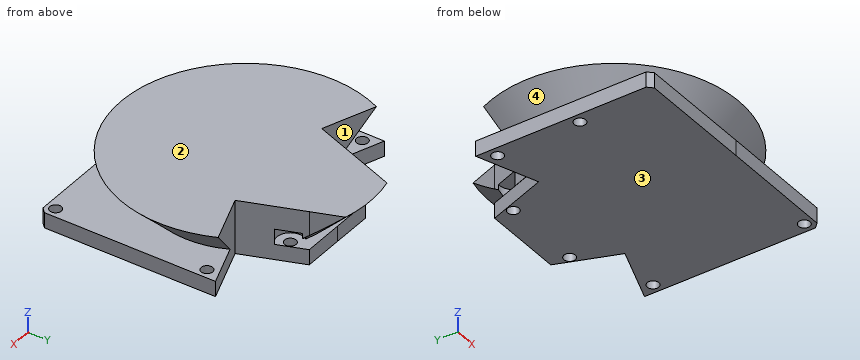
```python
from build123d import *

# Parameters (mm, degrees)
SKETCH9_R           = 1.4986
BOSS_EXTRUDE2_DEPTH = 4
SKETCH10_R          = 22.5
BOSS_EXTRUDE3_DEPTH = 10
BOSS_EXTRUDE3_DRAFT = -45
CUT_EXTRUDE1_DEPTH  = 10
SKETCH12_R          = 3.4986
CUT_EXTRUDE2_DEPTH  = 4


with BuildPart() as part:
    # Sketch9 → Boss-Extrude2 (new body)
    with BuildSketch(Plane.XY):
        Polygon((0, 45.894331692), (15.488494665, 40.257085472), (21.11579715, 55.718259441), (31.638563481, 55.718259441), (42.161245631, 55.760350338), (47.850347546, 40.321809178), (63.316169409, 46.020964031), (63.494666021, 1.396989332), (62.229756161, 0.121919512), (31.75, 0), (1.27, 0), (0, 1.27), align=None)
        with Locations((60.94984, 2.54)):
            Circle(SKETCH9_R, mode=Mode.SUBTRACT)
        with Locations((21.082, 50.8)):
            Circle(SKETCH9_R, mode=Mode.SUBTRACT)
        with Locations((2.54, 41.91)):
            Circle(SKETCH9_R, mode=Mode.SUBTRACT)
        with Locations(Location((60.792126991, 42.026504254, 0), (0, 0, 180))):
            Circle(SKETCH9_R, mode=Mode.SUBTRACT)
        with Locations(Location((42.214715469, 50.842265431, 0), (0, 0, 180))):
            Circle(SKETCH9_R, mode=Mode.SUBTRACT)
        with Locations((2.45872, 20.32)):
            Circle(SKETCH9_R, mode=Mode.SUBTRACT)
    extrude(amount=BOSS_EXTRUDE2_DEPTH)


with BuildPart() as boss_extrude3_tool:
    # Sketch10 → Boss-Extrude3 (with draft: the straight prism first)
    with BuildSketch(Plane.XY.offset(4)):
        with Locations((31.623, 31.75)):
            Circle(SKETCH10_R)
    extrude(amount=BOSS_EXTRUDE3_DEPTH)
    # Boss-Extrude3: the draft: its side faces are tilted about the plane it starts from
    boss_extrude3_sides = [boss_extrude3_tool.faces().sort_by_distance(p)[0] for p in [
        (9.123, 31.75, 9),
    ]]
    draft(boss_extrude3_sides, Plane.XY.offset(4), BOSS_EXTRUDE3_DRAFT)


with BuildPart() as part_1:
    add(part.part)

    # Boss-Extrude3: add boss_extrude3_tool
    add(boss_extrude3_tool.part)

    # Sketch11 → Cut-Extrude1 (cut)
    with BuildSketch(Plane.XY.offset(4)):
        Polygon((63.316169409, 46.020964031), (54.671905515, 69.478941389), (39.206083653, 63.779786536), (42.161245631, 55.760350338), (47.850347546, 40.321809178), align=None)
        Polygon((-0.039042446, 46.020964031), (15.426779416, 40.321809178), (21.115881332, 55.760350338), (24.071043309, 63.779786536), (8.605221447, 69.478941389), align=None)
    extrude(amount=CUT_EXTRUDE1_DEPTH, mode=Mode.SUBTRACT)

    # Sketch12 → Cut-Extrude2 (cut)
    with BuildSketch(Plane.XY.offset(4)):
        with Locations((21.062411493, 50.842265431)):
            Circle(SKETCH12_R)
        with Locations((42.214715469, 50.842265431)):
            Circle(SKETCH12_R)
    extrude(amount=CUT_EXTRUDE2_DEPTH, mode=Mode.SUBTRACT)


solid = part_1.part
```
Input: part model. Units: mm. Frame: model coordinates. Face numbers are marked on the shaded views. A direction names the side the tool comes from. Give positions to 0.01 mm unless a question says otherwise; leave off trailing zeros. Loops run counter-clockwise (first coordinate to the right, second up) from the corner with the lowest first, then second, coordinate; pieces in that order, holes last.
1) Section query A-A on z = 9.25. Return the cut outline in (x, y), and give its area (3 significant figures).
A:
outline: (6.53, 43.6) arc R27.75 ccw (long way) to (56.72, 43.59) - (47.85, 40.32) - (41.45, 57.7) arc R27.75 ccw to (21.84, 57.72) - (15.43, 40.32) - close
area: 2,190 mm2
2) Reachability of the marked faces 3 and 4 from +Z, -Z, +X, -X, +Y, -Y: full face, straight path, thin tool, end or side. Return the list, or none.
A:
face 3: -Z, +X, -X, +Y, -Y
face 4: none
3) Section query D-D on y = 2.54. Count the separate pieces of the cut face and the enclosed holes in it, and give its area (3 significant figures).
A:
separate pieces: 3
enclosed holes: 0
area: 304 mm2
4) Section query C-C on z = 1.5. Return the cut outline in (x, y).
A:
outline: (0, 1.27) - (1.27, 0) - (31.75, 0) - (62.23, 0.12) - (63.49, 1.4) - (63.32, 46.02) - (47.85, 40.32) - (42.16, 55.76) - (31.64, 55.72) - (21.12, 55.72) - (15.49, 40.26) - (0, 45.89) - close; hole circle Ø3 at (2.46, 20.32); hole circle Ø3 at (2.54, 41.91); hole circle Ø3 at (21.08, 50.8); hole circle Ø3 at (42.21, 50.84); hole circle Ø3 at (60.79, 42.03); hole circle Ø3 at (60.95, 2.54)
5) Mould query, pull axis X, two halves, no side actions, for the marked faces 1 and 2. Classes: released by +X, released by -X, zero draft, split by the parting line, or undercut.
A:
face 1: undercut
face 2: zero draft
6) Section query B-B on y = 31.75. Return the cut outline in (x, z), and give its area (3 significant figures).
A:
outline: (-0.88, 14) - (9.12, 4) - (0, 4) - (0, 0) - (63.37, 0) - (63.37, 4) - (54.12, 4) - (64.12, 14) - close
area: 803 mm2
7) Line query: L1, parallel to Y at x = 60, z = 1.5; L2, parallel to Z at x = 25, y = 8; L3, parallel to Y at x = 29, z = 0.5. Output: solid intervals per line, ascending.
A:
L1: y = 0.11 to 1.38, 3.7 to 40.75, 43.3 to 44.8
L2: z = 0 to 4, 6.16 to 14
L3: y = 0 to 55.72
8) Contact query for flat-ended pins moving along their axis: pin 1 (4.5 mm diameter, centred on x = 23.5, z = 3, fed in from -Y); pin 2 (2.5 mm diameter, centred on x = 2.54, y = 41.91, fed in from -Z); pin 3 (6 mm diameter, centred on x = 36.5, z = 4, fed in from +Y); pin 4 (2.5 mm diameter, centred on x = 60.95, y = 2.54, fed in from +Z). Output: stop coordinate, or through.
A:
pin 1: stops at y = 0
pin 2: stops at z = 11.06
pin 3: stops at y = 56.83
pin 4: passes through
